Geometry check sheet. Reference: the model listing, model coordinates, mm. A direction names the side the tool comes from. Coordinates: 2 decimals unless noted, no trailing zeros. Loops run counter-clockwise (first coordinate to the right, second up) from the corner with the lowest first, then second, coordinate; pieces in that order, holes last. Notation, with made-up numbers: (19.5, 29) - (39.5, 29) arc R35 ccw to (39.5, 65) - close; hole circle Ø10 at (75, 33.5). An arc over 180 degrees is marked (long way). Write item = value, one per line. Start each with the question number.
from build123d import *

# Parameters (mm, degrees)
SKETCH_219_W        = 218
SKETCH_219_H        = 134
SKETCH_219_W_2      = 198
SKETCH_219_H_2      = 114
EXTRUDE_2_DEPTH     = 16
SKETCH_2_W          = 126
SKETCH_2_H          = 12
CUT_EXTRUDE_1_DEPTH = 212
SKETCH_3_W          = 182
SKETCH_3_H          = 14.4
CUT_EXTRUDE_2_DEPTH = 134
SKETCH_4_R          = 1
CUT_EXTRUDE_3_DEPTH = 1.6
FILLET_1_R          = 3
FILLET_2_R          = 3
FILLET_3_R          = 3


with BuildPart() as part:
    # Sketch 219 → Бобышка-Вытянуть2 (new body)
    with BuildSketch(Plane(origin=(0, 0, 0), x_dir=(1, 0, 0), z_dir=(0, 1, 0))):
        Rectangle(SKETCH_219_W, SKETCH_219_H)
        Rectangle(SKETCH_219_W_2, SKETCH_219_H_2, mode=Mode.SUBTRACT)
    extrude(amount=EXTRUDE_2_DEPTH)

    # Эскиз2 → Вырез-Вытянуть1 (cut)
    with BuildSketch(Plane.ZY.offset(109)):
        with Locations((0, 7.6)):
            Rectangle(SKETCH_2_W, SKETCH_2_H)
    extrude(amount=-CUT_EXTRUDE_1_DEPTH, mode=Mode.SUBTRACT)

    # Эскиз3 → Вырез-Вытянуть2 (cut)
    with BuildSketch(Plane.XY.offset(67)):
        with Locations((0, 8.8)):
            Rectangle(SKETCH_3_W, SKETCH_3_H)
    extrude(amount=-CUT_EXTRUDE_2_DEPTH, mode=Mode.SUBTRACT)

    # Эскиз4 → Вырез-Вытянуть3 (cut)
    with BuildSketch(Plane(origin=(0, 1.6, 0), x_dir=(1, 0, 0), z_dir=(0, 1, 0))):
        with Locations(Location((-74.698916604, 62, 0), (0, 0, 270))):
            Circle(SKETCH_4_R)
        with Locations(Location((-74.698916604, -62, 0), (0, 0, 270))):
            Circle(SKETCH_4_R)
        with Locations(Location((74.698916604, -62, 0), (0, 0, 90))):
            Circle(SKETCH_4_R)
        with Locations(Location((74.698916604, 62, 0), (0, 0, 90))):
            Circle(SKETCH_4_R)
    extrude(amount=-CUT_EXTRUDE_3_DEPTH, mode=Mode.SUBTRACT)

    # Скругление1
    fillet_1_edges = [part.edges().sort_by_distance(p)[0] for p in [
        (109, 8, 67),
        (-109, 8, 67),
        (-109, 8, -67),
        (109, 8, -67),
    ]]
    fillet(fillet_1_edges, radius=FILLET_1_R)

    # Скругление2
    # the kernel refuses this fillet: 3 mm, written as the material it takes off along each edge
    with BuildSketch(Plane(origin=(-91, 16, -49.5), x_dir=(-1, 0, 0), z_dir=(0, 0, -1)), Plane(origin=(-91, 16, 74.5), x_dir=(-1, 0, 0), z_dir=(0, 0, -1))) as fillet_2_piece_1:
        with BuildLine():
            CenterArc((FILLET_2_R, -FILLET_2_R), FILLET_2_R, 90, 90)
            Line((0, -FILLET_2_R), (0, 0))
            Line((0, 0), (FILLET_2_R, 0))
        make_face()
    extrude(amount=25, mode=Mode.SUBTRACT)
    with BuildSketch(Plane(origin=(-83.651530772, 16, -57), x_dir=(0, 0, -1), z_dir=(-1, 0, 0)), Plane(origin=(-99, 16, 57), x_dir=(0, 0, 1), z_dir=(1, 0, 0))) as fillet_2_piece_2:
        with BuildLine():
            CenterArc((2.939387691, 3), FILLET_2_R, 191.536959033, 78.463040967)
            Line((0, 2.4), (0, 0))
            Line((0, 0), (2.939387691, 0))
        make_face()
    extrude(amount=15.348469228, mode=Mode.SUBTRACT)
    with BuildSketch(Plane(origin=(-99, 16, -57), x_dir=(-1, 0, 0), z_dir=(0, 0, 1))) as fillet_2_piece_3:
        with BuildLine():
            CenterArc((2.939387691, 3), FILLET_2_R, 191.536959033, 78.463040967)
            Line((0, 2.4), (0, 0))
            Line((0, 0), (2.939387691, 0))
        make_face()
    extrude(amount=114, mode=Mode.SUBTRACT)
    with BuildSketch(Plane(origin=(-106, 16, 67), x_dir=(0, -1, 0), z_dir=(1, 0, 0))) as fillet_2_piece_4:
        with BuildLine():
            CenterArc((FILLET_2_R, FILLET_2_R), FILLET_2_R, 180, 90)
            Line((0, FILLET_2_R), (0, 0))
            Line((0, 0), (FILLET_2_R, 0))
        make_face()
    extrude(amount=22.5, mode=Mode.SUBTRACT)
    with BuildSketch(Plane(origin=(-106, 16, 64), x_dir=(0, 0, 1), z_dir=(1, 0, 0))) as fillet_2_piece_5:
        with BuildLine():
            CenterArc((3 - FILLET_2_R, FILLET_2_R), FILLET_2_R, 270, 90)
            Line((3 - FILLET_2_R, 0), (3, 0))
            Line((3, 0), (3, FILLET_2_R))
        make_face()
    revolve(axis=Axis((-106, 16, 64), (0, -1, 0)), revolution_arc=90, mode=Mode.SUBTRACT)
    with BuildSketch(Plane(origin=(-109, 16, -64), x_dir=(1, 0, 0), z_dir=(0, 0, 1))) as fillet_2_piece_6:
        with BuildLine():
            CenterArc((FILLET_2_R, -FILLET_2_R), FILLET_2_R, 90, 90)
            Line((0, -FILLET_2_R), (0, 0))
            Line((0, 0), (FILLET_2_R, 0))
        make_face()
    extrude(amount=128, mode=Mode.SUBTRACT)
    with BuildSketch(Plane(origin=(-106, 16, -64), x_dir=(-1, 0, 0), z_dir=(0, 0, 1))) as fillet_2_piece_7:
        with BuildLine():
            CenterArc((3 - FILLET_2_R, FILLET_2_R), FILLET_2_R, 270, 90)
            Line((3, FILLET_2_R), (3, 0))
            Line((3, 0), (3 - FILLET_2_R, 0))
        make_face()
    revolve(axis=Axis((-106, 16, -64), (0, -1, 0)), revolution_arc=90, mode=Mode.SUBTRACT)
    with BuildSketch(Plane(origin=(-83.5, 16, -67), x_dir=(0, 0, 1), z_dir=(-1, 0, 0))) as fillet_2_piece_8:
        with BuildLine():
            CenterArc((FILLET_2_R, -FILLET_2_R), FILLET_2_R, 90, 90)
            Line((0, -FILLET_2_R), (0, 0))
            Line((0, 0), (FILLET_2_R, 0))
        make_face()
    extrude(amount=22.5, mode=Mode.SUBTRACT)
    with BuildSketch(Plane(origin=(-91, 16, -57), x_dir=(0, 0, -1), z_dir=(-1, 0, 0))) as fillet_2_piece_9a_section:
        with BuildLine():
            CenterArc((2.939387691, 3), FILLET_2_R, 191.536959033, 78.463040967)
            Line((0, 2.4), (0, 0))
            Line((0, 0), (2.939387691, 0))
        make_face()
    fillet_2_piece_9a = extrude(amount=15.348469228, mode=Mode.PRIVATE)
    fillet_2_piece_9a = split(fillet_2_piece_9a, bisect_by=Plane(origin=(-99, 16, -57), z_dir=(-1, 0, 0)), keep=Keep.TOP, mode=Mode.PRIVATE)
    with BuildSketch(Plane(origin=(-99, 16, -64.348469228), x_dir=(-1, 0, 0), z_dir=(0, 0, 1))) as fillet_2_piece_9b_section:
        with BuildLine():
            CenterArc((2.939387691, 3), FILLET_2_R, 191.536959033, 78.463040967)
            Line((0, 2.4), (0, 0))
            Line((0, 0), (2.939387691, 0))
        make_face()
    fillet_2_piece_9b = extrude(amount=121.348469228, mode=Mode.PRIVATE)
    fillet_2_piece_9b = split(fillet_2_piece_9b, bisect_by=Plane(origin=(-99, 16, -57), z_dir=(0, 0, -1)), keep=Keep.TOP, mode=Mode.PRIVATE)
    fillet_2_piece_9b = split(fillet_2_piece_9b, bisect_by=Plane(origin=(-99, 16, -63), z_dir=(0, 0, 1)), keep=Keep.TOP, mode=Mode.PRIVATE)
    fillet_2_piece_9 = fillet_2_piece_9a & fillet_2_piece_9b
    add(fillet_2_piece_9, mode=Mode.SUBTRACT)
    with BuildSketch(Plane(origin=(-106.348469228, 16, 57), x_dir=(0, 0, 1), z_dir=(1, 0, 0))) as fillet_2_piece_10a_section:
        with BuildLine():
            CenterArc((2.939387691, 3), FILLET_2_R, 191.536959033, 78.463040967)
            Line((0, 2.4), (0, 0))
            Line((0, 0), (2.939387691, 0))
        make_face()
    fillet_2_piece_10a = extrude(amount=15.348469228, mode=Mode.PRIVATE)
    fillet_2_piece_10a = split(fillet_2_piece_10a, bisect_by=Plane(origin=(-99, 16, 57), z_dir=(-1, 0, 0)), keep=Keep.TOP, mode=Mode.PRIVATE)
    with BuildSketch(Plane(origin=(-99, 16, -57), x_dir=(-1, 0, 0), z_dir=(0, 0, 1))) as fillet_2_piece_10b_section:
        with BuildLine():
            CenterArc((2.939387691, 3), FILLET_2_R, 191.536959033, 78.463040967)
            Line((0, 2.4), (0, 0))
            Line((0, 0), (2.939387691, 0))
        make_face()
    fillet_2_piece_10b = extrude(amount=121.348469228, mode=Mode.PRIVATE)
    fillet_2_piece_10b = split(fillet_2_piece_10b, bisect_by=Plane(origin=(-99, 16, 57), z_dir=(0, 0, 1)), keep=Keep.TOP, mode=Mode.PRIVATE)
    fillet_2_piece_10b = split(fillet_2_piece_10b, bisect_by=Plane(origin=(-99, 16, 63), z_dir=(0, 0, -1)), keep=Keep.TOP, mode=Mode.PRIVATE)
    fillet_2_piece_10 = fillet_2_piece_10a & fillet_2_piece_10b
    add(fillet_2_piece_10, mode=Mode.SUBTRACT)

    # Скругление3
    # the kernel refuses this fillet: 3 mm, written as the material it takes off along each edge
    with BuildSketch(Plane(origin=(106, 16, 64), x_dir=(0, 0, 1), z_dir=(-1, 0, 0))) as fillet_3_piece_1:
        with BuildLine():
            CenterArc((3 - FILLET_3_R, -FILLET_3_R), FILLET_3_R, 0, 90)
            Line((3, -FILLET_3_R), (3, 0))
            Line((3, 0), (3 - FILLET_3_R, 0))
        make_face()
    revolve(axis=Axis((106, 16, 64), (0, 1, 0)), revolution_arc=90, mode=Mode.SUBTRACT)
    with BuildSketch(Plane(origin=(83.5, 16, 67), x_dir=(0, -1, 0), z_dir=(1, 0, 0)), Plane(origin=(106, 16, -67), x_dir=(0, -1, 0), z_dir=(-1, 0, 0))) as fillet_3_piece_2:
        with BuildLine():
            CenterArc((FILLET_3_R, FILLET_3_R), FILLET_3_R, 180, 90)
            Line((0, FILLET_3_R), (0, 0))
            Line((0, 0), (FILLET_3_R, 0))
        make_face()
    extrude(amount=22.5, mode=Mode.SUBTRACT)
    with BuildSketch(Plane(origin=(91, 16, 74.5), x_dir=(0, -1, 0), z_dir=(0, 0, -1)), Plane(origin=(91, 16, -49.5), x_dir=(0, -1, 0), z_dir=(0, 0, -1))) as fillet_3_piece_3:
        with BuildLine():
            CenterArc((FILLET_3_R, -FILLET_3_R), FILLET_3_R, 90, 90)
            Line((0, -FILLET_3_R), (0, 0))
            Line((0, 0), (FILLET_3_R, 0))
        make_face()
    extrude(amount=25, mode=Mode.SUBTRACT)
    with BuildSketch(Plane(origin=(83.651530772, 16, 57), x_dir=(0, -1.0, 1.5720758028687117e-12), z_dir=(1, 0, 0)), Plane(origin=(99, 16, -57), x_dir=(0, -1.0, -1.5750363976010446e-12), z_dir=(-1, 0, 0))) as fillet_3_piece_4:
        with BuildLine():
            CenterArc((3, -2.939387691), FILLET_3_R, 101.536959033, 78.463040967)
            Line((0, -2.939387691), (0, 0))
            Line((0, 0), (2.4, 0))
        make_face()
    extrude(amount=15.348469228, mode=Mode.SUBTRACT)
    with BuildSketch(Plane(origin=(99, 16, 57), x_dir=(1.56911520813638e-12, -1.0, 0), z_dir=(0, 0, -1))) as fillet_3_piece_5:
        with BuildLine():
            CenterArc((3, -2.939387691), FILLET_3_R, 101.536959033, 78.463040967)
            Line((0, -2.939387691), (0, 0))
            Line((0, 0), (2.4, 0))
        make_face()
    extrude(amount=114, mode=Mode.SUBTRACT)
    with BuildSketch(Plane(origin=(106, 16, -64), x_dir=(1, 0, 0), z_dir=(0, 0, 1))) as fillet_3_piece_6:
        with BuildLine():
            CenterArc((3 - FILLET_3_R, -FILLET_3_R), FILLET_3_R, 0, 90)
            Line((3 - FILLET_3_R, 0), (3, 0))
            Line((3, 0), (3, -FILLET_3_R))
        make_face()
    revolve(axis=Axis((106, 16, -64), (0, 1, 0)), revolution_arc=90, mode=Mode.SUBTRACT)
    with BuildSketch(Plane(origin=(109, 16, 64), x_dir=(0, -1, 0), z_dir=(0, 0, -1))) as fillet_3_piece_7:
        with BuildLine():
            CenterArc((FILLET_3_R, FILLET_3_R), FILLET_3_R, 180, 90)
            Line((0, FILLET_3_R), (0, 0))
            Line((0, 0), (FILLET_3_R, 0))
        make_face()
    extrude(amount=128, mode=Mode.SUBTRACT)
    with BuildSketch(Plane(origin=(91, 16, 57), x_dir=(0, -1.0, 1.5720758028687117e-12), z_dir=(1, 0, 0))) as fillet_3_piece_8a_section:
        with BuildLine():
            CenterArc((3, -2.939387691), FILLET_3_R, 101.536959033, 78.463040967)
            Line((0, -2.939387691), (0, 0))
            Line((0, 0), (2.4, 0))
        make_face()
    fillet_3_piece_8a = extrude(amount=15.348469228, mode=Mode.PRIVATE)
    fillet_3_piece_8a = split(fillet_3_piece_8a, bisect_by=Plane(origin=(103, 16, 57), z_dir=(-1, 0, 0)), keep=Keep.TOP, mode=Mode.PRIVATE)
    fillet_3_piece_8a = split(fillet_3_piece_8a, bisect_by=Plane(origin=(99, 16, 57), z_dir=(1, 0, 0)), keep=Keep.TOP, mode=Mode.PRIVATE)
    with BuildSketch(Plane(origin=(99, 16, 64.348469228), x_dir=(1.56911520813638e-12, -1.0, 0), z_dir=(0, 0, -1))) as fillet_3_piece_8b_section:
        with BuildLine():
            CenterArc((3, -2.939387691), FILLET_3_R, 101.536959033, 78.463040967)
            Line((0, -2.939387691), (0, 0))
            Line((0, 0), (2.4, 0))
        make_face()
    fillet_3_piece_8b = extrude(amount=121.348469228, mode=Mode.PRIVATE)
    fillet_3_piece_8b = split(fillet_3_piece_8b, bisect_by=Plane(origin=(99, 16, 63), z_dir=(0, 0, -1)), keep=Keep.TOP, mode=Mode.PRIVATE)
    fillet_3_piece_8b = split(fillet_3_piece_8b, bisect_by=Plane(origin=(99, 16, 57), z_dir=(0, 0, 1)), keep=Keep.TOP, mode=Mode.PRIVATE)
    fillet_3_piece_8 = fillet_3_piece_8a & fillet_3_piece_8b
    add(fillet_3_piece_8, mode=Mode.SUBTRACT)
    with BuildSketch(Plane(origin=(99, 16, 57), x_dir=(1.56911520813638e-12, -1.0, 0), z_dir=(0, 0, -1))) as fillet_3_piece_9a_section:
        with BuildLine():
            CenterArc((3, -2.939387691), FILLET_3_R, 101.536959033, 78.463040967)
            Line((0, -2.939387691), (0, 0))
            Line((0, 0), (2.4, 0))
        make_face()
    fillet_3_piece_9a = extrude(amount=121.348469228, mode=Mode.PRIVATE)
    fillet_3_piece_9a = split(fillet_3_piece_9a, bisect_by=Plane(origin=(99, 16, -63), z_dir=(0, 0, 1)), keep=Keep.TOP, mode=Mode.PRIVATE)
    fillet_3_piece_9a = split(fillet_3_piece_9a, bisect_by=Plane(origin=(99, 16, -57), z_dir=(0, 0, -1)), keep=Keep.TOP, mode=Mode.PRIVATE)
    with BuildSketch(Plane(origin=(106.348469228, 16, -57), x_dir=(0, -1.0, -1.5750363976010446e-12), z_dir=(-1, 0, 0))) as fillet_3_piece_9b_section:
        with BuildLine():
            CenterArc((3, -2.939387691), FILLET_3_R, 101.536959033, 78.463040967)
            Line((0, -2.939387691), (0, 0))
            Line((0, 0), (2.4, 0))
        make_face()
    fillet_3_piece_9b = extrude(amount=15.348469228, mode=Mode.PRIVATE)
    fillet_3_piece_9b = split(fillet_3_piece_9b, bisect_by=Plane(origin=(103, 16, -57), z_dir=(-1, 0, 0)), keep=Keep.TOP, mode=Mode.PRIVATE)
    fillet_3_piece_9b = split(fillet_3_piece_9b, bisect_by=Plane(origin=(99, 16, -57), z_dir=(1, 0, 0)), keep=Keep.TOP, mode=Mode.PRIVATE)
    fillet_3_piece_9 = fillet_3_piece_9a & fillet_3_piece_9b
    add(fillet_3_piece_9, mode=Mode.SUBTRACT)


solid = part.part
(1) Tool access check on faces 5 (the face through (-19, 1.6, -60)), 6 (the face through (-91, 7, 65)), 7 (the face through (97, 8, -63)), 8 (the face through (103, 16, 0)). Record the directions out of +Z, -Z, +X, -X, +Y, -Y that give a thin tool (end or side, any length) a straight path to the whole face; none if there is none.
(2) Sectioned sample at B-B on y = 10.25. Enter the section's corners in (x, z), plus the area to 3 significant figures.
(3) Depth check by flat-ended pin: pin 1 (1 mm diameter, centred on y = 9, z = -38, fed in from -X). Enter the tip coordinate at first touch or a pass-through.
(4) Scan lines: line 1 (X direction, y = 0.9, z = 62); line 2 (X direction, y = 1.25, z = -45); line 3 (Z direction, x = 70.5, y = 1). Record each from-to range of solid material in increasing order.
(5) Sectioned sample at A-A on z = -42. Enter the section's corners in (x, y), plus the area to 3 significant figures.
(6) Draft check along Z on faces 1 (the face through (-100, 8, 63)), 2 (the face through (0, 1, 67)), 3 (the face through (91, 7, 65)), 4 (the face through (0, 1, -67)). Enter one of: pulls with the +Z half, pulls with the -Z half, needs draft (parallel to the pull), parting line crosses it, or undercut.
Working result:
q1.face_5 = none
q1.face_6 = +Z, -Z, +Y
q1.face_7 = -X
q1.face_8 = +Z, -Z, +X, -X, +Y
q2.outline = (-109, -64) arc R3 ccw to (-106, -67) - (-91, -67) - (-91, -63) - (-109, -63) - close; (-109, 63) - (-91, 63) - (-91, 67) - (-106, 67) arc R3 ccw to (-109, 64) - close; (91, -67) - (106, -67) arc R3 ccw to (109, -64) - (109, 64) arc R3 ccw to (106, 67) - (91, 67) - (91, 63) - (103, 63) - (103, -63) - (91, -63) - close
q2.area = 1,040 mm2
q3.pin_1 = 103
q4.line_1 = -109 to -75.7, -73.7 to 73.7, 75.7 to 109
q4.line_2 = -109 to -99, 99 to 109
q4.line_3 = -67 to -57, 57 to 67
q5.outline = (-109, 0) - (-99, 0) - (-99, 1.6) - (-109, 1.6) - close; (-108.94, 13.6) - (-99, 13.6) arc R3 ccw to (-101.94, 16) - (-106, 16) arc R3 ccw to start; (99, 0) - (109, 0) - (109, 13) arc R3 ccw to (106, 16) - (101.94, 16) arc R3 ccw to (99, 13.6) - (103, 13.6) - (103, 1.6) - (99, 1.6) - close
q5.area = 145 mm2
q6.face_1 = undercut
q6.face_2 = pulls with the +Z half
q6.face_3 = needs draft
q6.face_4 = pulls with the -Z half
